Geometry: final body of the model. Coordinates: model frame, mm. A direction names the side the tool comes from. Round coordinates to 2 decimals unless told otherwise and drop trailing zeros. Loops run counter-clockwise (first coordinate to the right, second up) from the corner with the lowest first, then second, coordinate; pieces in that order, holes last. Notation, with made-up numbers: (2.5, -10.5) - (40.5, -10.5) arc R37 cw to (40.5, 28.5) - close; hole circle Ø5 at (34.25, 8). An arc over 180 degrees is marked (long way). Write item = value, one per line. Start each with the question number.
Item 1: Section C-C (y = -5.5). Return loops of the section in (x, z), plus the area to 3 significant figures.
Item 2: Draft query along X for faces 3 (the cylindrical face through (21.537, -0.986, -20.202)), 4 (the cylindrical face through (26.68, -1.01, 24.4)), 5 (the flat face through (0, -1, 25)), 6 (the cylindrical face through (-18.69, -0.99, 20.83)). Return one class per face: pulls with the +X half, pulls with the -X half, needs draft (parallel to the pull), parting line crosses it, or undercut.
Item 3: Section D-D (y = -20). Return loops of the section in (x, z), plus the area to 3 significant figures.
Item 4: Section B-B (z = -20). Return loops of the section in (x, y).
Item 5: First-contact query: pin 1 (4 mm diameter, centred on x = -20, z = 20, fed in from +Y); pin 2 (6 mm diameter, centred on x = 9, z = -5, fed in from -Y); pin 3 (2.5 mm diameter, centred on x = -20, z = -20, fed in from +Y); pin 4 (1.6 mm diameter, centred on y = -0.5, z = 12.5, fed in from +X). Flat tips, straight axial feed; report the tip coordinate or a pass-through.
Item 6: Section A-A (x = 20). Return loops of the section in (y, z).
Item 7: Line query: line 1 (Z direction, x = -28.95, y = -20); line 2 (X direction, y = -8, z = -9); line 3 (Y direction, x = 22, z = -19). Output: solid intervals per line, ascending. Write a range as from..to.
Item 8: Access query for faces 1 (the cylindrical face through (29.26, -20.35, -16.22)), 2 (the flat face through (-28.25, -20, -9)). Directions: +Z, -Z, +X, -X, +Y, -Y. A direction counts if a zero-diameter tool reaches every point of the face in a straight line with its end or side. Return the directions, or none.
from build123d import *

# Parameters (mm, degrees)
SKETCH1_W               = 54.5
SKETCH1_H               = 50
BASE_FLANGE1_DEPTH      = 2
EDGE_FLANGE1_DEPTH      = 31
EDGE_FLANGE1_BEND_DEPTH = 31
SKETCH12_R              = 1.55
CUT_EXTRUDE1_DEPTH      = 54.935725637
SKETCH13_R              = 1.6
CUT_EXTRUDE2_DEPTH      = 76.194747157
BREAK_CORNER1_START     = -30.25
BREAK_CORNER1_DEPTH     = 60.5
BREAK_CORNER1_START_2   = -2
BREAK_CORNER1_2_DEPTH   = 2


# Read off the part's stored shape, not the designer's step: Break-Corner1
# Sheet-metal steps are written as plain solids
with BuildPart() as part:
    # Sketch1 → Base-Flange1 (new body)
    with BuildSketch(Plane(origin=(0, 0, 0), x_dir=(1, 0, 0), z_dir=(0, 1, 0))):
        Rectangle(SKETCH1_W, SKETCH1_H)
    extrude(amount=-BASE_FLANGE1_DEPTH)

    # Edge-Flange1 section (across the edge) → Edge-Flange1 (add)
    with BuildSketch(Plane(origin=(28.25, -2, -25), x_dir=(-1, 0, 0), z_dir=(0, 0, 1))):
        with BuildLine():
            Line((-2, 1), (-2, 35))
            Line((-2, 35), (0, 35))
            Line((0, 35), (0, 1))
            ThreePointArc((0, 1), (0.292893219, 0.292893219), (1, 0))
            Line((1, 0), (1, -2))
            ThreePointArc((1, -2), (-1.121320344, -1.121320344), (-2, 1))
        make_face()
    extrude(amount=EDGE_FLANGE1_DEPTH)

    # Edge-Flange1 section 2 (across the edge) → Edge-Flange1 bend (add)
    with BuildSketch(Plane(origin=(-28.25, -2, 6), x_dir=(1, 0, 0), z_dir=(0, 0, -1))):
        with BuildLine():
            Line((-2, 1), (-2, 35))
            Line((-2, 35), (0, 35))
            Line((0, 35), (0, 1))
            ThreePointArc((0, 1), (0.292893219, 0.292893219), (1, 0))
            Line((1, 0), (1, -2))
            ThreePointArc((1, -2), (-1.121320344, -1.121320344), (-2, 1))
        make_face()
    extrude(amount=EDGE_FLANGE1_BEND_DEPTH)

    # Sketch12 → Cut-Extrude1 (cut, through all)
    with BuildSketch(Plane(origin=(0, 0, 0), x_dir=(1, 0, 0), z_dir=(0, 1, 0))):
        with Locations(Location((-20, 20, 0), (0, 0, 270))):
            Circle(SKETCH12_R)
        with Locations(Location((20, 20, 0), (0, 0, 270))):
            Circle(SKETCH12_R)
        with Locations(Location((20, -20, 0), (0, 0, 270))):
            Circle(SKETCH12_R)
        with Locations(Location((-20, -20, 0), (0, 0, 270))):
            Circle(SKETCH12_R)
    extrude(amount=-CUT_EXTRUDE1_DEPTH, mode=Mode.SUBTRACT)

    # Sketch13 → Cut-Extrude2 (cut, through all)
    with BuildSketch(Plane(origin=(30.25, 0, 0), x_dir=(0, 0, -1), z_dir=(1, 0, 0))):
        with Locations(Location((14.66, -20, 0), (0, 0, 90))):
            Circle(SKETCH13_R)
        with Locations(Location((4.33, -20, 0), (0, 0, 90))):
            Circle(SKETCH13_R)
    extrude(amount=-CUT_EXTRUDE2_DEPTH, mode=Mode.SUBTRACT)

    # Break-Corner1 outline → Break-Corner1 (cut)
    with BuildSketch(Plane.YZ.offset(BREAK_CORNER1_START)):
        with BuildLine():
            ThreePointArc((-35, -25), (-36.414213562, -24.414213562), (-37, -23))
            Line((-37, -23), (-37, -25))
            Line((-37, -25), (-35, -25))
        make_face()
        with BuildLine():
            ThreePointArc((-37, 4), (-36.414213562, 5.414213562), (-35, 6))
            Line((-35, 6), (-37, 6))
            Line((-37, 6), (-37, 4))
        make_face()
    extrude(amount=BREAK_CORNER1_DEPTH, mode=Mode.SUBTRACT)

    # Break-Corner1 2 outline → Break-Corner1 2 (cut)
    with BuildSketch(Plane(origin=(0, 0, 0), x_dir=(1, 0, 0), z_dir=(0, 1, 0)).offset(BREAK_CORNER1_START_2)):
        with BuildLine():
            Line((-27.25, -25), (-25.25, -25))
            ThreePointArc((-25.25, -25), (-26.664213562, -24.414213562), (-27.25, -23))
            Line((-27.25, -23), (-27.25, -25))
        make_face()
        with BuildLine():
            ThreePointArc((27.25, -23), (26.664213562, -24.414213562), (25.25, -25))
            Line((25.25, -25), (27.25, -25))
            Line((27.25, -25), (27.25, -23))
        make_face()
    extrude(amount=BREAK_CORNER1_2_DEPTH, mode=Mode.SUBTRACT)


solid = part.part
Taken from the geometry:
q1.outline = (-30.25, -25) - (-28.25, -25) - (-28.25, 6) - (-30.25, 6) - close; (28.25, -25) - (30.25, -25) - (30.25, 6) - (28.25, 6) - close
q1.area = 124 mm^2
q2.face_3 = undercut
q2.face_4 = pulls with the +X half
q2.face_5 = needs draft
q2.face_6 = undercut
q3.outline = (-30.25, -25) - (-28.25, -25) - (-28.25, -16.26) - (-30.25, -16.26) - close; (-30.25, -13.06) - (-28.25, -13.06) - (-28.25, -5.93) - (-30.25, -5.93) - close; (-30.25, -2.73) - (-28.25, -2.73) - (-28.25, 6) - (-30.25, 6) - close; (28.25, -25) - (30.25, -25) - (30.25, -16.26) - (28.25, -16.26) - close; (28.25, -13.06) - (30.25, -13.06) - (30.25, -5.93) - (28.25, -5.93) - close; (28.25, -2.73) - (30.25, -2.73) - (30.25, 6) - (28.25, 6) - close
q3.area = 98.4 mm^2
q4.outline = (-30.25, -37) - (-28.25, -37) - (-28.25, -3) arc R1 cw to (-27.25, -2) - (-21.55, -2) - (-21.55, 0) - (-27.25, 0) arc R3 ccw to (-30.25, -3) - close; (-18.45, -2) - (18.45, -2) - (18.45, 0) - (-18.45, 0) - close; (21.55, -2) - (27.25, -2) arc R1 cw to (28.25, -3) - (28.25, -37) - (30.25, -37) - (30.25, -3) arc R3 ccw to (27.25, 0) - (21.55, 0) - close
q5.pin_1 = 0
q5.pin_2 = -2
q5.pin_3 = through
q5.pin_4 = 27.25
q6.outline = (-2, -25) - (0, -25) - (0, -21.55) - (-2, -21.55) - close; (-2, -18.45) - (0, -18.45) - (0, 18.45) - (-2, 18.45) - close; (-2, 21.55) - (0, 21.55) - (0, 25) - (-2, 25) - close
q7.line_1 = -25..-16.26, -13.06..-5.93, -2.73..6
q7.line_2 = -30.25..-28.25, 28.25..30.25
q7.line_3 = -2..0
q8.face_1 = +X, -X
q8.face_2 = +Z, -Z, -Y
